Geometry check sheet. Reference: the model listing, model coordinates, mm. Face numbers are marked on the shaded views. Round coordinates to 2 decimals unless told otherwise and drop trailing zeros. Write each loop counter-clockwise with the first axis right and the second up, starting at its lowest first coordinate (ties: lowest second). Pieces come first, ordered by that corner, then holes.
from build123d import *

# Parameters (mm, degrees)
SKETCH1_R           = 3
BOSS_EXTRUDE1_DEPTH = 2.5


with BuildPart() as part:
    # Sketch1 → Boss-Extrude1 (new body)
    with BuildSketch(Plane(origin=(0, 0, 0), x_dir=(1, 0, 0), z_dir=(0, 1, 0))):
        with BuildLine():
            Line((16.504384769, 67.001942846), (13.497620534, 67.780107201))
            Line((13.497620534, 67.780107201), (7.724071328, 57.579565356))
            add(Edge.make_bspline(
                [(-0.09847484, 11.22942621), (11.417322618, 26.843615689), (14.193248849, 43.730948361), (7.724071328, 57.579565356)],
                knots=[0.117374877, 0.117374877, 0.117374877, 0.117374877, 0.726153686, 0.726153686, 0.726153686, 0.726153686], degree=3))
            ThreePointArc((-0.09847484, 11.22942621), (-0.351961708, 10.90026492), (-0.618902028, 10.581916664))
            ThreePointArc((-0.618902028, 10.581916664), (-1.844722259, -10.438246969), (4.208359749, 9.728808161))
            ThreePointArc((4.208359749, 9.728808161), (4.214374117, 13.50532277), (5.497341127, 17.05723696))
            add(Edge.make_bspline(
                [(5.497341127, 17.05723696), (6.247224749, 18.369564751), (6.949389536, 19.705033958), (7.925084618, 21.74584693), (8.237367579, 22.432397455), (8.834853314, 23.818631134), (9.120431061, 24.519332655), (10.471450422, 28.041849379), (11.3095387, 30.920313304), (12.007053004, 34.605583669), (12.12890822, 35.347032839), (12.335497702, 36.839176051), (12.420373432, 37.591640588), (12.615035285, 39.850848786), (12.664547894, 41.35101651), (12.566324851, 45.833161956), (12.175786709, 48.797076432), (11.415069816, 51.733451528)],
                knots=[0, 0, 0, 0, 0.125, 0.125, 0.1875, 0.1875, 0.25, 0.25, 0.5, 0.5, 0.5625, 0.5625, 0.625, 0.625, 0.75, 0.75, 1, 1, 1, 1], degree=3))
            ThreePointArc((11.415069816, 51.733451528), (11.157464025, 55.926562312), (12.490570585, 59.910450575))
            Line((12.490570585, 59.910450575), (16.504384769, 67.001942846))
        make_face()
        with Locations(Location((0, 0, 0), (0, 0, 270))):
            Circle(SKETCH1_R, mode=Mode.SUBTRACT)
    extrude(amount=BOSS_EXTRUDE1_DEPTH)


solid = part.part
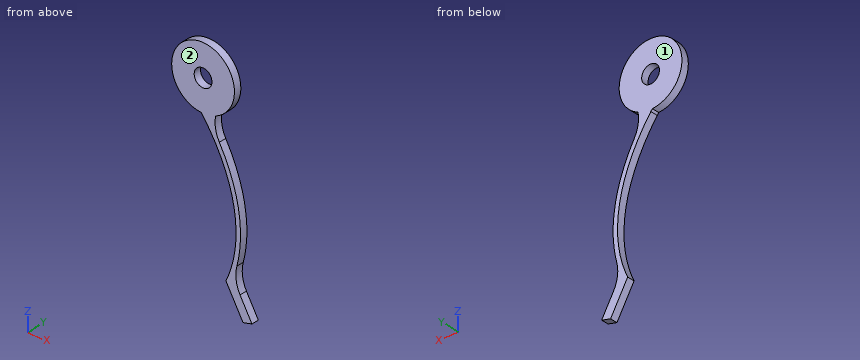
1. Release check for a two-part mould opening along Y. For the marked faces 1 and 2 record: +Y half, -Y half, draft (parallel to the pull), parting line (faces both ways), or undercut.
2. Scan lines: line 1 along X through (y, z) = (0.8, 0); line 2 along Z through (x, y) = (0.75, 1); line 3 along Z through (x, y) = (0.5, 2.3). Record each from-to range of solid material in increasing order.
3. Depth check by flat-ended pin: pin 1 Ø7 at (x, z) = (0, 0) entering from +Y; pin 2 Ø1 at (x, y) = (7.5, 1.5) entering from -Z; pin 3 Ø2 at (x, z) = (1, 0.5) entering from -Y. Enter the tip coordinate at first touch or a pass-through.
4. Section check A-A (z = 0). Record the cut outline in (x, y).
5. Section check B-B (x = -6.25). Record the cut outline in (y, z), plus the area to 3 significant figures.
Results below:
1. face 1: +Y half
1. face 2: -Y half
2. line 1: x = -10.6 to -3, 3 to 10.6
2. line 2: z = -12.4 to -2.9, 2.9 to 10.57
2. line 3: z = -12.05 to -2.96, 2.96 to 10.59
3. pin 1: stops at y = 2.5
3. pin 2: stops at z = -58.07
3. pin 3: passes through
4. outline: (-10.6, 0) - (-3, 0) - (-3, 2.5) - (-10.6, 2.5) - close; (3, 0) - (10.6, 0) - (10.6, 2.5) - (3, 2.5) - close
5. outline: (0, -8.56) - (2.5, -8.56) - (2.5, 8.56) - (0, 8.56) - close
5. area: 42.8 mm2
